Can you work these out from the model? Positions are in its coordinate system, mm. Face numbers are marked on the shaded views. Coordinates: 2 decimals unless noted, no trailing zeros. Order: outer loops, then holes, each group sorted by start corner. A loop starts at its lowest first (then second) coordinate and runs counter-clockwise, first axis right, second up. Notation, with made-up numbers: M 36,31 L 69,31 A8 ccw 69,37 Z; hole C 67,54 d9. An arc over 180 degrees is marked long. Answer as a JSON object with one key per item and string values.
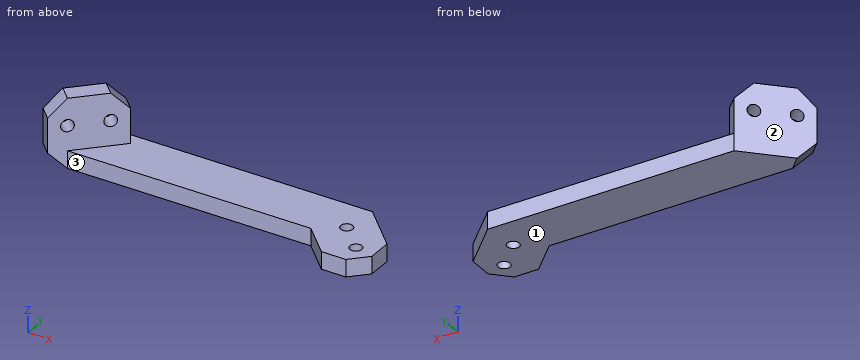
from build123d import *

# Parameters (mm, degrees)
F0_W      = 82
F0_H      = 17
F1_DEPTH  = 5.75
F2_W      = 24.0416305603
F2_H      = 23
F3_DEPTH  = 5.75
F4_R      = 2
F5_DEPTH  = 25
F6_SIZE   = 5.75
F8_DEPTH  = 5.75
F9_R      = 2
F10_DEPTH = 25
F11_SIZE  = 5.75


with BuildPart() as f1:
    # F0 (on Top) → F1 (new body)
    with BuildSketch(Plane.XY):
        Rectangle(F0_W, F0_H)
        Polygon((41, 8.5), (41, -8.5), (58, -8.5), align=None)
        Polygon((-58, -8.5), (-41, -8.5), (-41, 8.5), align=None)
    extrude(amount=F1_DEPTH)

    # F2 (on face) → F3 (join)
    with BuildSketch(Plane(origin=(-24.75, 24.75, 0), x_dir=(-0.7071067812, -0.7071067812, 0), z_dir=(-0.7071067812, 0.7071067812, 0))):
        with Locations((35.0017856687, 11.5)):
            Rectangle(F2_W, F2_H)
    extrude(amount=-F3_DEPTH)

    # F4 (on face) → F5 (cut)
    with BuildSketch(Plane(origin=(-24.75, 24.75, 0), x_dir=(-0.7071067812, -0.7071067812, 0), z_dir=(-0.7071067812, 0.7071067812, 0))):
        with Locations((28.7309703886, 14)):
            Circle(F4_R)
        with Locations((41.2726009489, 14)):
            Circle(F4_R)
    extrude(amount=-F5_DEPTH, mode=Mode.SUBTRACT)

    # F6
    f6_edges = [f1.edges().sort_by_distance(p)[0] for p in [
        (-55.967068, -10.532932, 23),
        (-38.967068, 6.467068, 23),
        (-55.967068, -10.532932, 0),
    ]]
    chamfer(f6_edges, length=F6_SIZE)

    # F7 (on face) → F8 (join)
    with BuildSketch(Plane.XY.offset(5.75)):
        Polygon((58, -8.5), (41, 8.5), (28.3015151902, -5.6715728753), (31.1299423149, -8.5), align=None)
        Polygon((44.5649711575, -21.9350288425), (58, -8.5), (31.1299423149, -8.5), align=None)
    extrude(amount=-F8_DEPTH)

    # F9 (on face) → F10 (cut)
    with BuildSketch(Plane.XY.offset(5.75)):
        with Locations((47.5701749775, -10.7980970389)):
            Circle(F9_R)
        with Locations((39.4384469939, -2.6663690552)):
            Circle(F9_R)
    extrude(amount=-F10_DEPTH, mode=Mode.SUBTRACT)

    # F11
    f11_edges = [f1.edges().sort_by_distance(p)[0] for p in [
        (44.564971, -21.935029, 2.875),
        (58, -8.5, 2.875),
    ]]
    chamfer(f11_edges, length=F11_SIZE)


solid = f1.part
Item 1: I want a section at B-B, the plane x = -14.5. Write out the boundary of the cut face in (y, z).
Answers follow:
{"outline": "M -8.5,0 L 8.5,0 L 8.5,5.75 L -8.5,5.75 Z"}
Item 2: I'm going to push flat-ended pins straight in: pin 1 (3 mm diameter, centred on y = -5, z = 20, fed in from +X); pin 2 (8 mm diameter, centred on x = 22.5, y = 1, fed in from +Z); pin 3 (6.5 mm diameter, centred on x = 6, z = 2, fed in from -Y). Where does each tip first touch, or does it pass through?
Answers follow:
{"pin 1": "stops at x = -44.87", "pin 2": "stops at z = 5.75", "pin 3": "stops at y = -8.5"}
Item 3: If we mould it in two halves opening along X, with no side actions, what happens to the marked faces 1, 2 and 3? For each: pulls with the +X half, pulls with the -X half, needs draft (parallel to the pull), parting line crosses it, or undercut.
Answers follow:
{"face 1": "needs draft", "face 2": "pulls with the -X half", "face 3": "undercut"}
Item 4: I want a section at C-C, the plane y = -14.75. Write out the boundary of the cut face in (x, z).
Answers follow:
{"outline": "M 37.38,0 L 51.75,0 L 51.75,5.75 L 37.38,5.75 Z"}
Item 5: Please list where these lines run through material, in increasing order: line 1 (Z direction, x = -33, y = 1.75); line 2 (X direction, y = -3.25, z = 2.25); line 3 (X direction, y = -2, z = 3.5).
Answers follow:
{"line 1": "z = 0 to 5.75", "line 2": "x = -52.75 to 37.53, 41.35 to 52.75", "line 3": "x = -51.5 to 37.55, 41.32 to 51.5"}
Item 6: I want a section at A-A, the plane z = 4.75. Write out the boundary of the cut face in (x, y).
Answers follow:
{"outline": "M -57.29,-7.79 L -53.23,-11.86 L -49.87,-8.5 L 31.13,-8.5 L 40.5,-17.87 L 48.63,-17.87 L 53.93,-12.57 L 53.93,-4.43 L 41,8.5 L -41,8.5 Z; hole C 39.44,-2.67 d4; hole C 47.57,-10.8 d4"}
